Answer from the drawing. Dimensions are ordinates in mm from the lowest x, y and z of the part. Coordinates: 2 decimals unless noted, no trailing zeros. Order: outer loops, then holes, each group sorted by start corner. A loop starts at its lowest first (then second) coordinate and runs counter-clockwise, first axis right, second up. Notation, with made-up numbers: M 20.5,11.25 L 55.5,11.25 A14 cw 55.5,18.25 Z; hole C -1,33 d5. An arc over 180 degrees is marked long. Write each question's results on one line, items separated by ' | '.
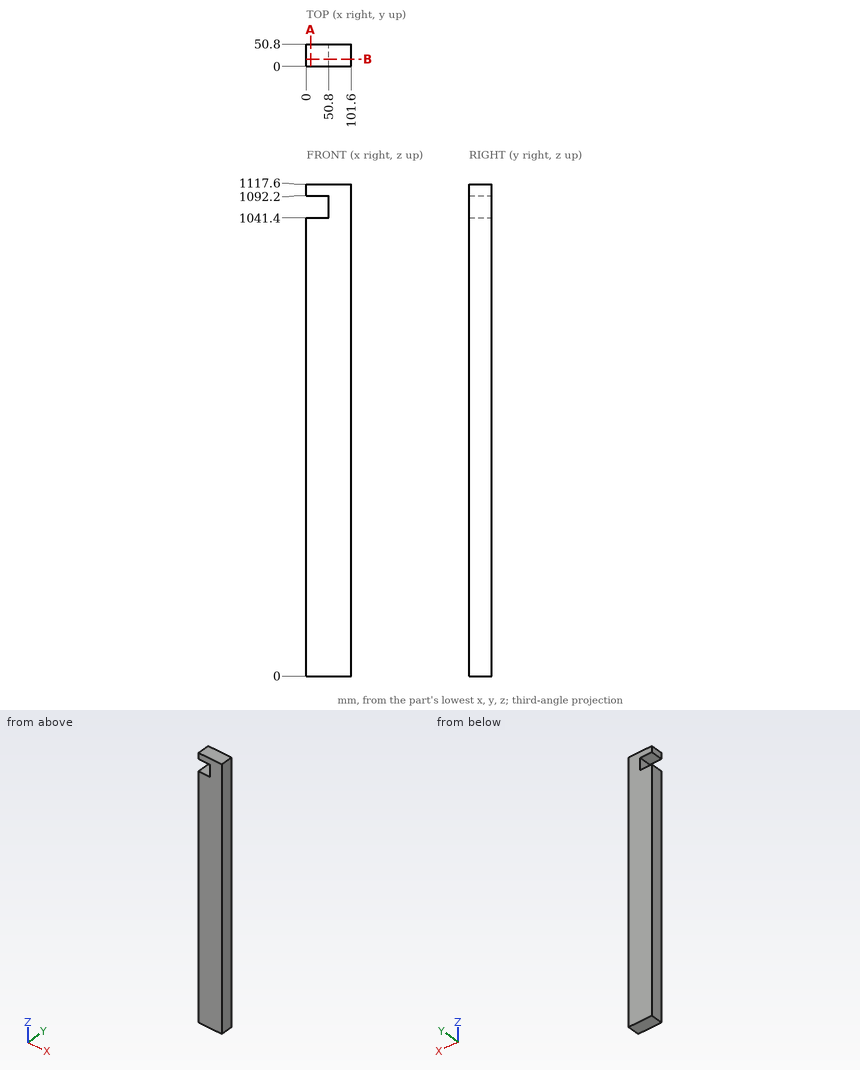
(1) Straight lines are drawn through the part: line 1 (Z direction, x = 48.5, y = 30.5); line 2 (X direction, y = 33, z = 1068). For each, find the intervals that lie inside material, in ascending order.
Conclusion:
line 1: 0 to 1041.4, 1092.2 to 1117.6 | line 2: 50.8 to 101.6
(2) Given pin 1 (15 mm diameter, centred on y = 14.5, z = 1061.5, fed in from -X), flat-ended and moving along its own axis, determine where the tip first touches the part or whether it passes through.
Conclusion:
pin 1: x = 50.8
(3) The part is cut by section A-A, the plane x = 9.5. Write down the section's boundary in (y, z), then the cut area to 3 significant figures.
Conclusion:
outline: M 0,0 L 50.8,0 L 50.8,1041.4 L 0,1041.4 Z; M 0,1092.2 L 50.8,1092.2 L 50.8,1117.6 L 0,1117.6 Z | area: 54,200 mm²
(4) The part is cut by section B-B, the plane y = 16.5. Write down the section's boundary in (x, z), then the cut area to 3 significant figures.
Conclusion:
outline: M 0,0 L 101.6,0 L 101.6,1117.6 L 0,1117.6 L 0,1092.2 L 50.8,1092.2 L 50.8,1041.4 L 0,1041.4 Z | area: 111,000 mm²
